For this review, use the dimensioned drawing (mm, ordinates from the lowest corner) and the shaded views. Give positions to 0.01 mm unless a question says otherwise; leave off trailing zeros. Order: outer loops, then holes, each group sorted by start corner. A loop starts at its lowest first (then second) coordinate and runs counter-clockwise, first axis right, second up. Notation, with made-up numbers: (49, 4.25) - (53, 4.25) arc R16 ccw to (53, 20.25) - close; hole circle Ø10 at (-35, -23). An arc over 180 degrees is marked (long way). Use a Markdown table: item, result. Add a question column.
1) We need section B-B on z = 12. Write out the cut boundary in (x, y), then the cut area to 3 significant figures.
2) We need section C-C on x = 59. Write out the cut boundary in (y, z).
3) We need section A-A on y = 68. Write out the cut boundary in (x, z).
4) Wall thickness on L1, parallel to Y at x = 57, z = 32.5; L2, parallel to X at y = 63.5, z = 13; L3, parallel to X at y = 61, z = 12: over which ranges is each line inside the solid? List them lowest first.
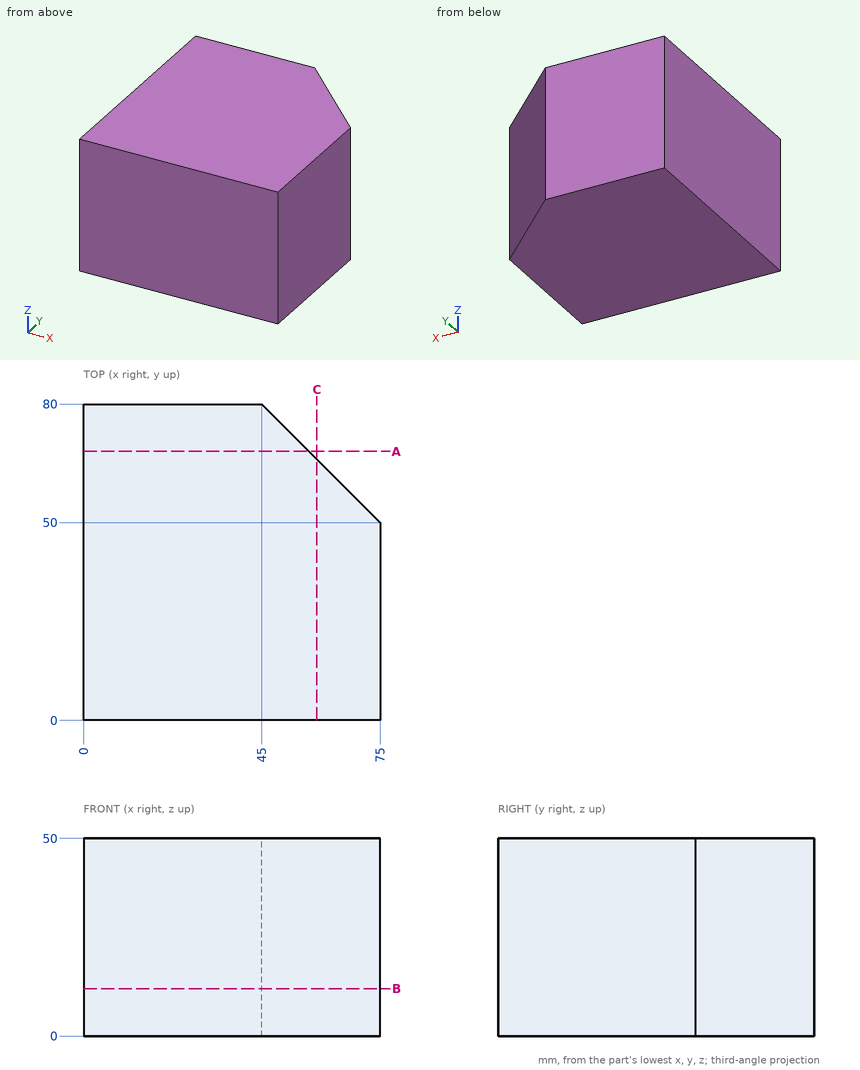
Checked values:
| question | item | result |
|---|---|---|
| 1 | outline | (0, 0) - (75, 0) - (75, 50) - (45, 80) - (0, 80) - close |
| 1 | area | 5,550 mm² |
| 2 | outline | (0, 0) - (66, 0) - (66, 50) - (0, 50) - close |
| 3 | outline | (0, 0) - (57, 0) - (57, 50) - (0, 50) - close |
| 4 | L1 | 0 to 68 |
| 4 | L2 | 0 to 61.5 |
| 4 | L3 | 0 to 64 |
